Part model, mm, in its own coordinate system. A direction names the side the tool comes from. Give positions to 0.01 mm unless a question says otherwise; leave off trailing zeros. Write each loop counter-clockwise with the first axis right and the second up, starting at its lowest first coordinate (ties: lowest second). Pieces come first, ordered by that corner, then holes. Notation, with made-up numbers: (29, 86) - (56, 86) arc R16 ccw to (56, 106) - close; hole circle Ø8 at (-19.5, -3). An arc over 180 degrees is marked (long way). Answer in a Markdown table with one row per item. Add a question column.
1. Band-saw the part on A-A on z = -2. Write the cut outline in (x, y), plus the area to 3 significant figures.
2. Band-saw the part on C-C on z = 3.25. Write the cut outline in (x, y), plus the area to 3 significant figures.
3. Pull direction Z, two halves, no side cores. Call faces 1 (the flat face through (0, 0, -6)), 2 (the conical face through (5.013, 2.079, 3.388)), 3 (the flat face through (0, 0, 0)): released by +Z, released by -Z, zero draft, split by the parting line, or undercut.
4. Probe line 1 along Z through (x, y) = (1.25, 2); line 2 along Y through (x, z) = (2.25, 5.75); line 3 along Z through (x, y) = (-2.75, 3.5). List the from-to ranges inside material, lowest first.
5. Which spindle directions (+Z, -Z, +X, -X, +Y, -Y) get a long thin tool onto all of the face, cutting with end or side? Do faces 4 (the conical face through (4.69, -1.48, 3.41)), 5 (the cylindrical face through (-0.07, 4.99, 5.11)), 6 (the cylindrical face through (-3, 0, -3)). Say none if no direction does.
6. Band-saw the part on B-B on x = 0. Write the cut outline in (y, z).
7. Drop flat-ended pins along their axis: pin 1 Ø6 at (x, z) = (-4, 4.5) entering from +Y; pin 2 Ø5 at (x, z) = (-3, 1) entering from +Y. Give the stop position or say it passes through.
```python
from build123d import *

# Parameters (mm, degrees)
F2_R     = 0.5
F3_DEPTH = 25


with BuildPart() as f1:
    # F0 (on Front) → F1 (revolve)
    with BuildSketch(Plane.XZ):
        with BuildLine():
            Line((5.420953, 0), (0, 0))
            Line((0, 0), (0, -0.5))
            Line((0, -0.5), (0, -6))
            Line((0, -6), (3, -6))
            Line((3, -6), (3, -0.5))
            Line((3, -0.5), (5.884191, -0.5))
            ThreePointArc((5.884191, -0.5), (5.959879, -0.465356), (5.983123, -0.385427))
            Line((5.983123, -0.385427), (5.083987, 5.718595))
            ThreePointArc((5.083987, 5.718595), (4.580334, 6.635318), (3.6, 7))
            Line((3.6, 7), (0, 7))
            Line((0, 7), (0, 6.5))
            Line((0, 6.5), (3.6, 6.5))
            ThreePointArc((3.6, 6.5), (4.253556, 6.256878), (4.589324, 5.64573))
            Line((4.589324, 5.64573), (5.420953, 0))
        make_face()
    revolve(axis=Axis((0, 0, 3.25), (0, 0, -1)))

    # F2 (on Front) → F3 (cut)
    with BuildSketch(Plane.XZ):
        with Locations((0, 4.614573)):
            Circle(F2_R)
    extrude(amount=-F3_DEPTH, mode=Mode.SUBTRACT)


solid = f1.part
```
Values:
| question | item | result |
|---|---|---|
| 1 | outline | circle Ø6 at (0, 0) |
| 1 | area | 28.3 mm² |
| 2 | outline | circle Ø10.9 at (0, 0); hole circle Ø9.88 at (0, 0) |
| 2 | area | 16.5 mm² |
| 3 | face 1 | released by -Z |
| 3 | face 2 | released by +Z |
| 3 | face 3 | undercut |
| 4 | line 1 | z = -6 to 0, 6.5 to 7 |
| 4 | line 2 | y = -4.55 to -3.98, 3.98 to 4.55 |
| 4 | line 3 | z = -0.5 to 0, 6.02 to 6.74 |
| 5 | face 4 | none |
| 5 | face 5 | +Y |
| 5 | face 6 | -Z |
| 6 | outline | (-5.98, -0.39) arc R0.1 ccw to (-5.88, -0.5) - (-3, -0.5) - (-3, -6) - (3, -6) - (3, -0.5) - (5.88, -0.5) arc R0.1 ccw to (5.98, -0.39) - (5.32, 4.11) - (4.81, 4.11) - (5.42, 0) - (-5.42, 0) - (-4.59, 5.65) arc R1 cw to (-3.6, 6.5) - (3.6, 6.5) arc R1 cw to (4.59, 5.65) - (4.67, 5.11) - (5.17, 5.11) - (5.08, 5.72) arc R1.5 ccw to (3.6, 7) - (-3.6, 7) arc R1.5 ccw to (-5.08, 5.72) - close |
| 7 | pin 1 | stops at y = 5.3 |
| 7 | pin 2 | stops at y = 5.91 |
